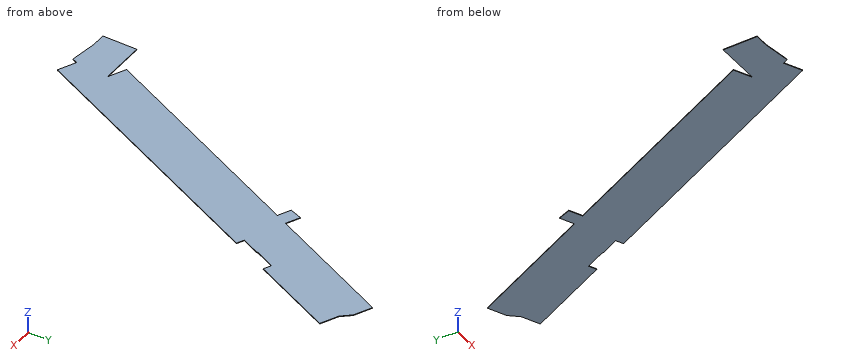
```python
from build123d import *

# Parameters (mm, degrees)
EXTRUDE_1_DEPTH = 1
EXTRUDE_2_DEPTH = 2


with BuildPart() as part:
    # 草图1 → 拉伸1 (new body)
    with BuildSketch(Plane.XY.offset(49.5)):
        Polygon((1390.105050596, -579.075609045), (1377.377505434, -564.434243188), (1350.188271823, -551.755695336), (1258.268799894, -748.877639017), (1237.099840045, -739.006390924), (1239.746814184, -733.845622773), (1226.4, -727), (1213.4, -757.7), (1226.746814184, -764.545622773), (1230.039181278, -758.126541077), (1249.684280108, -767.287201107), (1198.420684959, -877.222335675), (1183.121903884, -910.030677565), (1170.274308727, -937.582434291), (1150.664821383, -979.63511561), (1135.45056396, -1012.262195943), (1122.349397846, -1040.357737342), (1107.895853295, -1071.353463658), (1090.610766389, -1108.421452148), (1117.8, -1121.1), (1046.2, -1121.1), (1046.2, -1174.6), (1068.2, -1174.6), (1110, -1180.474606891), (1113.845826182, -1172.227206029), (1141.035059793, -1184.905753881), (1329.933624158, -779.811475326), (1318.78530378, -774.612928158), (1332.080038523, -746.102277496), (1331.173730736, -745.679659234), (1345.965369897, -713.958886688), (1357.747371128, -719.45292409), (1417.294284207, -591.754156897), align=None)
    extrude(amount=-EXTRUDE_1_DEPTH)

    # 草图2 → 拉伸2 (cut)
    with BuildSketch(Plane.XY.offset(49.5)):
        Polygon((1239.746814184, -733.845622773), (1226.4, -727), (1213.4, -757.7), (1226.746814184, -764.545622773), (1230.039181278, -758.126541078), (1237.099840045, -739.006390924), align=None)
    extrude(amount=-EXTRUDE_2_DEPTH, mode=Mode.SUBTRACT)


solid = part.part
```
Geometry check sheet. Reference: the model listing, model coordinates, mm. Coordinates: 2 decimals unless noted, no trailing zeros. Order: outer loops, then holes, each group sorted by start corner. A loop starts at its lowest first (then second) coordinate and runs counter-clockwise, first axis right, second up.
Item 1: Section check B-B (x = 1265). Enter the section's corners in (y, z).
Item 2: Section check C-C (y = -651.5). Enter the section's corners in (x, z).
Item 3: Scan lines: line 1 along Y through (x, z) = (1112.5, 49.4); line 2 along Y through (x, z) = (1113, 48.7); line 3 along Y through (x, z) = (1353, 49). Record each from-to range of solid material in increasing order.
Item 4: Section check A-A (z = 49.3). Enter the section's corners in (x, y), plus the area to 3 significant figures.
Item 5: Depth check by flat-ended pin: pin 1 (0.5 mm diameter, centred on x = 1093.5, z = 49, fed in from +Y). Enter the tip coordinate at first touch or a pass-through.
Check sheet entries:
1. outline: (-919.06, 48.5) - (-734.44, 48.5) - (-734.44, 49.5) - (-919.06, 49.5) - close
2. outline: (1303.68, 48.5) - (1389.43, 48.5) - (1389.43, 49.5) - (1303.68, 49.5) - close
3. line 1: y = -1175.11 to -1121.1, -1118.63 to -1061.48
3. line 2: y = -1174.04 to -1121.1, -1118.86 to -1060.41
3. line 3: y = -717.24 to -553.07
4. outline: (1046.2, -1174.6) - (1068.2, -1174.6) - (1110, -1180.47) - (1113.85, -1172.23) - (1141.04, -1184.91) - (1329.93, -779.81) - (1318.79, -774.61) - (1332.08, -746.1) - (1331.17, -745.68) - (1345.97, -713.96) - (1357.75, -719.45) - (1417.29, -591.75) - (1390.11, -579.08) - (1377.38, -564.43) - (1350.19, -551.76) - (1258.27, -748.88) - (1237.1, -739.01) - (1230.04, -758.13) - (1249.68, -767.29) - (1090.61, -1108.42) - (1117.8, -1121.1) - (1046.2, -1121.1) - close
4. area: 52,900 mm2
5. pin 1: stops at y = -1101.69
